from build123d import *

# Parameters (mm, degrees)
BOSS_EXTRUDE1_DEPTH = 27
BOSS_EXTRUDE2_DEPTH = 2
BOSS_EXTRUDE3_DEPTH = 1
SKETCH4_R           = 1.5
CUT_EXTRUDE1_DEPTH  = 42.701318924
SKETCH5_R           = 1.5
CUT_EXTRUDE2_DEPTH  = 10


with BuildPart() as part:
    # Sketch1 → Boss-Extrude1 (new, symmetric)
    with BuildSketch(Plane.XY):
        with BuildLine():
            Line((-31, 3), (-23.539392014, 3))
            ThreePointArc((-23.539392014, 3), (-14, 10), (-4.460607986, 3))
            Line((-4.460607986, 3), (4.460607986, 3))
            ThreePointArc((4.460607986, 3), (14, 10), (23.539392014, 3))
            Line((23.539392014, 3), (31, 3))
            Line((31, 3), (31, 0))
            Line((31, 0), (21.5, 0))
            ThreePointArc((21.5, 0), (14, 7.5), (6.5, 0))
            Line((6.5, 0), (-6.5, 0))
            ThreePointArc((-6.5, 0), (-14, 7.5), (-21.5, 0))
            Line((-21.5, 0), (-31, 0))
            Line((-31, 0), (-31, 3))
        make_face()
    extrude(amount=BOSS_EXTRUDE1_DEPTH, both=True)

    # Sketch2 → Boss-Extrude2 (add)
    with BuildSketch(Plane.XY.offset(27)):
        with BuildLine():
            Line((-22, 0), (-21, 0))
            ThreePointArc((-21, 0), (-14, 7), (-7, 0))
            Line((-7, 0), (-6, 0))
            ThreePointArc((-6, 0), (-14, 8), (-22, 0))
        make_face()
        with BuildLine():
            Line((21, 0), (22, 0))
            ThreePointArc((22, 0), (14, 8), (6, 0))
            Line((6, 0), (7, 0))
            ThreePointArc((7, 0), (14, 7), (21, 0))
        make_face()
    boss_extrude2 = extrude(amount=-BOSS_EXTRUDE2_DEPTH)

    # Mirror1: Boss-Extrude2 across plane
    add(boss_extrude2.mirror(Plane.XY))

    # Sketch3 → Boss-Extrude3 (add, symmetric)
    with BuildSketch(Plane.XY):
        with BuildLine():
            Line((-22, 0), (-21, 0))
            ThreePointArc((-21, 0), (-14, 7), (-7, 0))
            Line((-7, 0), (-6, 0))
            ThreePointArc((-6, 0), (-14, 8), (-22, 0))
        make_face()
        with BuildLine():
            Line((6, 0), (7, 0))
            ThreePointArc((7, 0), (14, 7), (21, 0))
            Line((21, 0), (22, 0))
            ThreePointArc((22, 0), (14, 8), (6, 0))
        make_face()
    extrude(amount=BOSS_EXTRUDE3_DEPTH, both=True)

    # Sketch4 → Cut-Extrude1 (cut, through all)
    with BuildSketch(Plane(origin=(0, 3, 0), x_dir=(1, 0, 0), z_dir=(0, 1, 0))):
        with Locations(Location((-27, 23, 0), (0, 0, 270))):
            Circle(SKETCH4_R)
        with Locations(Location((-27, -23, 0), (0, 0, 270))):
            Circle(SKETCH4_R)
        with Locations(Location((27, -23, 0), (0, 0, 270))):
            Circle(SKETCH4_R)
        with Locations(Location((27, 23, 0), (0, 0, 270))):
            Circle(SKETCH4_R)
        with Locations(Location((0, 0, 0), (0, 0, 270))):
            Circle(SKETCH4_R)
    extrude(amount=-CUT_EXTRUDE1_DEPTH, mode=Mode.SUBTRACT)

    # Sketch5 → Cut-Extrude2 (cut)
    with BuildSketch(Plane(origin=(0, 3, 0), x_dir=(1, 0, 0), z_dir=(0, 1, 0))):
        with Locations(Location((27, 5, 0), (0, 0, 270))):
            Circle(SKETCH5_R)
        with Locations(Location((27, -5, 0), (0, 0, 270))):
            Circle(SKETCH5_R)
    extrude(amount=-CUT_EXTRUDE2_DEPTH, mode=Mode.SUBTRACT)


solid = part.part
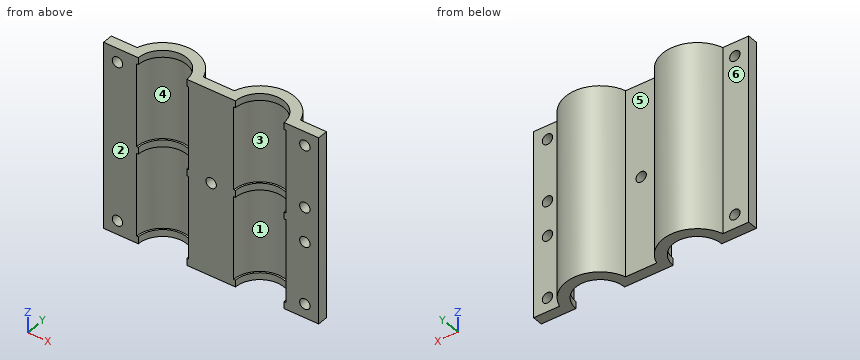
Verification items for the finished model (mm, model axes). Face numbers are marked on the shaded views. A direction names the side the tool comes from. Round coordinates to 2 decimals unless told otherwise and drop trailing zeros. Order: outer loops, then holes, each group sorted by start corner. A loop starts at its lowest first (then second) coordinate and runs counter-clockwise, first axis right, second up.
1. Thickness scan on L1, parallel to Z at x = -7, y = 2.25; L2, parallel to X at y = 1.4, z = -5; L3, parallel to X at y = 4, z = -9.5. Record the ranges inside material, lowest first.
Final values:
L1: z = -27 to -25, -1 to 1, 25 to 27
L2: x = -31 to -21.37, -6.63 to 6.63, 21.37 to 25.5, 28.5 to 31
L3: x = -23.17 to -20.34, -7.66 to -4.83, 4.83 to 7.66, 20.34 to 23.17
2. Go/stop test with flat-tipped pins: P1, Ø8, axis at x = -28.5, z = -10.5, coming from the +Y side; P2, Ø1.5, axis at x = -4.5, z = 4.5, coming from the +Y side. Record where each tip stops, or that it passes through.
Final values:
P1: stops at y = 3
P2: stops at y = 4.84
3. Section check D-D on z = -23. Record the cut outline in (x, y).
Final values:
outline: (-31, 0) - (-28.5, 0) - (-28.5, 3) - (-31, 3) - close; (-25.5, 0) - (-21.5, 0) arc R7.5 cw to (-6.5, 0) - (6.5, 0) arc R7.5 cw to (21.5, 0) - (25.5, 0) - (25.5, 3) - (23.54, 3) arc R10 ccw to (4.46, 3) - (-4.46, 3) arc R10 ccw to (-23.54, 3) - (-25.5, 3) - close; (28.5, 0) - (31, 0) - (31, 3) - (28.5, 3) - close
4. Section check B-B on x = -27. Record the cut outline in (y, z).
Final values:
outline: (0, -27) - (3, -27) - (3, -24.5) - (0, -24.5) - close; (0, -21.5) - (3, -21.5) - (3, 21.5) - (0, 21.5) - close; (0, 24.5) - (3, 24.5) - (3, 27) - (0, 27) - close
5. Access from +Z, -Z, +X, -X, +Y, -Y to the whole of each face (thin tool, end or side, straight path). Record for the marked faces 4, 5 and 6.
Final values:
face 4: -Y
face 5: +Z, -Z, +Y
face 6: +Z, -Z, -X, +Y
6. Section check A-A on z = 0. Record the cut outline in (x, y).
Final values:
outline: (-31, 0) - (-21, 0) arc R7 cw to (-7, 0) - (-1.5, 0) - (-1.5, 3) - (-4.46, 3) arc R10 ccw to (-23.54, 3) - (-31, 3) - close; (1.5, 0) - (7, 0) arc R7 cw to (21, 0) - (31, 0) - (31, 3) - (23.54, 3) arc R10 ccw to (4.46, 3) - (1.5, 3) - close
7. Section check C-C on x = 0. Record the cut outline in (y, z).
Final values:
outline: (0, -27) - (3, -27) - (3, -1.5) - (0, -1.5) - close; (0, 1.5) - (3, 1.5) - (3, 27) - (0, 27) - close
8. Release check for a two-part mould opening along Z. For the marked faces 1, 2 and 3 record: +Z half, -Z half, draft (parallel to the pull), parting line (faces both ways), or undercut.
Final values:
face 1: undercut
face 2: draft
face 3: undercut
